The listing builds one solid part. Answer for the finished solid, in the listing's coordinates (mm). A direction names the side the tool comes from. Round coordinates to 2 decimals unless told otherwise and drop trailing zeros. Order: outer loops, then holes, each group sorted by start corner. A loop starts at its lowest first (then second) coordinate and runs counter-clockwise, first axis right, second up. Notation, with made-up numbers: M 71.25,65.5 L 92.25,65.5 A23 cw 92.25,82.5 Z; hole C 21.25,46 d9. An arc over 180 degrees is marked long. Put each result on its own line as item: value. Start each with the question number.
1. Which of the six approach directions +Z, -Z, +X, -X, +Y, -Y give full straight-line access (tool end or side, diameter ignored) to faces 1 (the face through (102.5, -8.9, 46.6)), 2 (the face through (49, -16.5, 0)), 3 (the face through (49, 0, 17.5))?
2. The part is cut by section D-D (z = 22). Give the vertices of the cut face in (x, y).
3. The part is cut by section B-B (z = 43.5). Give the vertices of the cut face in (x, y), then the cut area to 3 significant figures.
4. Consider line 1 (Y direction, x = 76, z = -7); line 2 (X direction, y = 15.5, z = 10). Determine where each line is inside the solid, lowest interval first.
5. The mould has two halves that part along Z. Classify faces 4 (the face through (100, -0.4, 32.6)), 5 (the face through (52, 0, -17.5)), 6 (the face through (49, 0, -16.5)): +Z half, -Z half, draft (parallel to the pull), parting line (faces both ways), or undercut.
6. The part is cut by section A-A (x = 36). Give the vertices of the cut face in (y, z), then the cut area to 3 significant figures.
7. Each of these flat-tipped pins is pushed along its axis until it touches: pin 1 Ø2 at (x, y) = (87.5, -19) entering from -Z; pin 2 Ø10 at (x, y) = (94, 7) entering from +Z; pin 3 Ø3 at (x, z) = (37.5, 17) entering from -Y; pin 4 Ø10 at (x, z) = (54.5, 4.5) entering from +Y. Where does it stop, or does it pass through?
8. The part is cut by section C-C (z = 2). Give the vertices of the cut face in (x, y), then the cut area to 3 significant figures.
from build123d import *

# Parameters (mm, degrees)
F0_W     = 35
F0_H     = 35
F0_W_2   = 33
F0_H_2   = 33
F1_DEPTH = 100
F3_DEPTH = 5


with BuildPart() as f1:
    # F0 (on Right) → F1 (new body)
    with BuildSketch(Plane.YZ):
        Rectangle(F0_W, F0_H)
        Rectangle(F0_W_2, F0_H_2, mode=Mode.SUBTRACT)
    extrude(amount=F1_DEPTH)

    # F2 (on face) → F3 (join)
    with BuildSketch(Plane.YZ.offset(100)):
        with BuildLine():
            Line((-17.5, 17.5), (-17.5, -17.5))
            Line((-17.5, -17.5), (17.5, -17.5))
            Line((17.5, -17.5), (17.5, 17.5))
            Line((17.5, 17.5), (30.365003, 39.782839))
            ThreePointArc((30.365003, 39.782839), (30.365003, 44.782839), (26.034876, 47.282839))
            Line((26.034876, 47.282839), (11.421628, 47.282839))
            ThreePointArc((11.421628, 47.282839), (8.921628, 46.612966), (7.0915, 44.782839))
            Line((7.0915, 44.782839), (0, 32.5))
            Line((0, 32.5), (-7.0915, 44.782839))
            ThreePointArc((-7.0915, 44.782839), (-8.921628, 46.612966), (-11.421628, 47.282839))
            Line((-11.421628, 47.282839), (-26.034876, 47.282839))
            ThreePointArc((-26.034876, 47.282839), (-30.365003, 44.782839), (-30.365003, 39.782839))
            Line((-30.365003, 39.782839), (-17.5, 17.5))
        make_face()
    extrude(amount=F3_DEPTH)


solid = f1.part
Resolved:
1. face 1: +Z, +X, -X
1. face 2: -X
1. face 3: +Z, -X, +Y, -Y
2. outline: M 100,-20.1 L 105,-20.1 L 105,20.1 L 100,20.1 Z
3. outline: M 100,-30.88 L 105,-30.88 L 105,-6.35 L 100,-6.35 Z; M 100,6.35 L 105,6.35 L 105,30.88 L 100,30.88 Z
3. area: 245 mm2
4. line 1: -17.5 to -16.5, 16.5 to 17.5
4. line 2: 100 to 105
5. face 4: draft
5. face 5: -Z half
5. face 6: undercut
6. outline: M -17.5,-17.5 L 17.5,-17.5 L 17.5,17.5 L -17.5,17.5 Z; hole M -16.5,-16.5 L 16.5,-16.5 L 16.5,16.5 L -16.5,16.5 Z
6. area: 136 mm2
7. pin 1: through
7. pin 2: z = 17.5
7. pin 3: y = -17.5
7. pin 4: y = 17.5
8. outline: M 0,-17.5 L 105,-17.5 L 105,17.5 L 0,17.5 L 0,16.5 L 100,16.5 L 100,-16.5 L 0,-16.5 Z
8. area: 375 mm2
